Could you check a few things on this model? Use its own coordinates, in mm. A direction names the side the tool comes from. Give positions to 0.01 mm unless a question says otherwise; leave off trailing zeros. Order: outer loops, then holes, each group sorted by start corner. A loop starts at its lowest first (then second) coordinate and runs counter-clockwise, first axis right, second up. Notation, with made-up numbers: (-25.75, 11) -> (22.25, 11) arc R18 cw to (22.25, 24) -> close; hole circle Ø4 at (35.25, 51). An arc over 180 degrees is marked (long way). One line per item, written item: value.
```python
from build123d import *

# Parameters (mm, degrees)
SKETCH_1_R      = 2.5
EXTRUDE_1_DEPTH = 300


with BuildPart() as part:
    # 草图1 → 凸台-拉伸1 (new body)
    with BuildSketch(Plane.XY):
        Polygon((-20, 20), (-13.1, 20), (-13.1, 18.4), (-15.5, 18.4), (-15.5, 17.104298633), (-12.797022805, 13.9), (-7.202977195, 13.9), (-4.5, 17.104298633), (-4.5, 18.4), (-6.9, 18.4), (-6.9, 20), (0, 20), (0, 13.1), (-1.6, 13.1), (-1.6, 15.5), (-2.895701367, 15.5), (-6.1, 12.797022805), (-6.1, 7.202977195), (-2.895701367, 4.5), (-1.6, 4.5), (-1.6, 6.9), (0, 6.9), (0, 0), (-6.9, 0), (-6.9, 1.6), (-4.5, 1.6), (-4.5, 2.895701367), (-7.202977195, 6.1), (-12.797022805, 6.1), (-15.5, 2.895701367), (-15.5, 1.6), (-13.1, 1.6), (-13.1, 0), (-20, 0), (-20, 6.9), (-18.4, 6.9), (-18.4, 4.5), (-17.104298633, 4.5), (-13.9, 7.202977195), (-13.9, 12.797022805), (-17.104298633, 15.5), (-18.4, 15.5), (-18.4, 13.1), (-20, 13.1), align=None)
        with Locations((-10, 10)):
            Circle(SKETCH_1_R, mode=Mode.SUBTRACT)
    extrude(amount=EXTRUDE_1_DEPTH)


solid = part.part
```
1) If I drill on line 1 along X through (y, z) = (2.75, 142); line 2 along Y through (x, z) = (-19, 214); line 3 along Y through (x, z) = (-18.25, 78), over which ranges is the centre line in solid material (lowest first)?
Answer below:
line 1: x = -20 to -15.5, -4.5 to 0
line 2: y = 0 to 6.9, 13.1 to 20
line 3: y = 0 to 4.5, 15.5 to 20
2) Suppose I cut it at A-A, the plane x = -10. Write out the boundary of the cut face in (y, z), then the cut area to 3 significant figures.
Answer below:
outline: (6.1, 0) -> (7.5, 0) -> (7.5, 300) -> (6.1, 300) -> close; (12.5, 0) -> (13.9, 0) -> (13.9, 300) -> (12.5, 300) -> close
area: 840 mm2
3) For faces 5 (the flat face through (-13.9, 10, 148)), 6 (the flat face through (-8, 12, 0)), 7 (the flat face through (-6.1, 10, 148)), which set-ups out of +Z, -Z, +X, -X, +Y, -Y let a thin tool reach every point of the face, with its end or its side?
Answer below:
face 5: +Z, -Z, -X
face 6: -Z, +X, -X, +Y, -Y
face 7: +Z, -Z, +X
4) For P1, Ø3, axis at x = -9.5, z = 103, coming from the -Y side; P2, Ø1, axis at y = 7.5, z = 122, coming from the +X side, each with a flat end and sliding along its axis, tell me the tip position at first contact or that it passes through.
Answer below:
P1: stops at y = 6.1
P2: stops at x = -5.86
5) We'd pull the mould along X, two halves only. Please class faces 1 (the flat face through (-10, 6.1, 148)), 2 (the flat face through (0, 17, 148)), 3 (the flat face through (-20, 17, 148)), 4 (the flat face through (-10, 13.9, 148)): +X half, -X half, draft (parallel to the pull), parting line (faces both ways), or undercut.
Answer below:
face 1: undercut
face 2: +X half
face 3: -X half
face 4: undercut
6) Suppose I cut it at B-B, the plane y = 10. Write out the boundary of the cut face in (x, z), then the cut area to 3 significant figures.
Answer below:
outline: (-13.9, 0) -> (-12.5, 0) -> (-12.5, 300) -> (-13.9, 300) -> close; (-7.5, 0) -> (-6.1, 0) -> (-6.1, 300) -> (-7.5, 300) -> close
area: 840 mm2
